from build123d import *

# Parameters (mm, degrees)
F0_W     = 40
F0_H     = 40
F1_DEPTH = 10
F2_T     = -1
F3_R     = 1.25
F4_DEPTH = 10
F5_DEPTH = 25
F6_DEPTH = 25
F7_W     = 11
F7_H     = 1
F7_W_2   = 1
F7_H_2   = 11
F8_DEPTH = 6.5


with BuildPart() as f1:
    # F0 (on Top) → F1 (new body)
    with BuildSketch(Plane.XY):
        Rectangle(F0_W, F0_H)
    extrude(amount=F1_DEPTH)

    # F2
    f2_openings = [f1.faces().sort_by_distance(p)[0] for p in [
        (0, 0, 10),
    ]]
    offset(amount=F2_T, openings=f2_openings)

    # F3 (on face) → F4 (join)
    with BuildSketch(Plane.XY):
        Polygon((-20, -8.4495466982), (-20, -20), (-10.1382084124, -20), align=None)
        with Locations((-17.6, -17.6)):
            Circle(F3_R, mode=Mode.SUBTRACT)
        Polygon((20, -8.4495466982), (10.1382084124, -20), (20, -20), align=None)
        with Locations((17.6, -17.6)):
            Circle(F3_R, mode=Mode.SUBTRACT)
        Polygon((-20, 20), (-20, 8.4495466982), (-10.1382084124, 20), align=None)
        with Locations((-17.6, 17.6)):
            Circle(F3_R, mode=Mode.SUBTRACT)
        Polygon((20, 20), (10.1382084124, 20), (20, 8.4495466982), align=None)
        with Locations((17.6, 17.6)):
            Circle(F3_R, mode=Mode.SUBTRACT)
    extrude(amount=F4_DEPTH)

    # F3 (on face) → F5 (cut)
    with BuildSketch(Plane.XY):
        with Locations((-17.6, -17.6)):
            Circle(F3_R)
        with Locations((17.6, -17.6)):
            Circle(F3_R)
        with Locations((17.6, 17.6)):
            Circle(F3_R)
        with Locations((-17.6, 17.6)):
            Circle(F3_R)
    extrude(amount=F5_DEPTH, mode=Mode.SUBTRACT)

    # F6 (cut): a face of the model
    f6_faces = [f1.faces().sort_by_distance(p)[0] for p in [
        (0, 0, 1),
    ]]
    extrude(f6_faces, amount=-F6_DEPTH, mode=Mode.SUBTRACT)

    # F7 (on face) → F8 (cut)
    with BuildSketch(Plane.XY.offset(10)):
        with Locations((0, 19.5)):
            Rectangle(F7_W, F7_H)
        with Locations((0, -19.5)):
            Rectangle(F7_W, F7_H)
        with Locations((-19.5, 0)):
            Rectangle(F7_W_2, F7_H_2)
        with Locations((19.5, 0)):
            Rectangle(F7_W_2, F7_H_2)
    extrude(amount=-F8_DEPTH, mode=Mode.SUBTRACT)


solid = f1.part
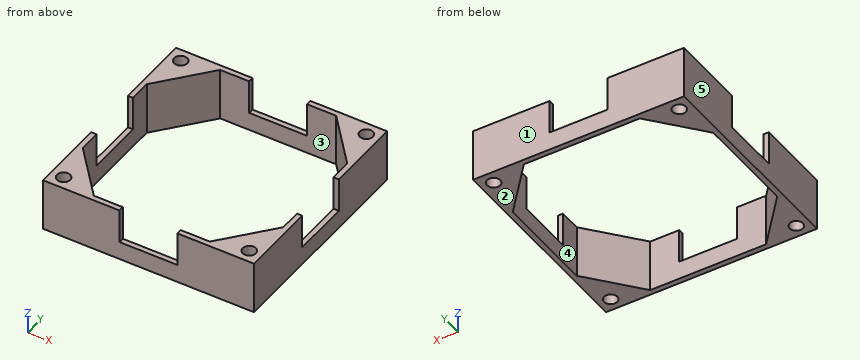
For this review, take the finished solid that the model builds, in its own axes (mm). Face numbers are marked on the shaded views. A direction names the side the tool comes from. Round coordinates to 2 decimals unless told otherwise and drop trailing zeros. Order: outer loops, then holes, each group sorted by start corner. A loop starts at its lowest first (then second) coordinate and runs counter-clockwise, first axis right, second up. Notation, with made-up numbers: M 38,-7 L 42,-7 A14 cw 42,10 Z; hole C 55.25,-28.5 d3. An arc over 180 degrees is marked long. Use a Markdown table: item, result. Add a question column.
Item 1: To check wall thickness, follow line 1 along X through (y, z) = (-3, 1.25); line 2 along Y through (x, z) = (-17, 6). State the ranges of each line that lie inside material, in increasing order.
Item 2: Add section D-D, the plane x = 17.6. Give the boundary of the cut face in (y, z), then the cut area to 3 significant figures.
Item 3: Mouldability with a two-part tool opening along Y and no side actions: class the marked faces 1, 2 and 3 as released by +Y, released by -Y, zero draft, split by the parting line, or undercut.
Item 4: Tool access review of the marked faces 4 and 5: name each direction out of +Z, -Z, +X, -X, +Y, -Y from which nothing blocks a thin tool from reaching the whole face with its end or side.
Item 5: Insertion check: pin 1 (1.1 mm diameter, centred on x = 2.5, y = -19.5, fed in from +Z); pin 2 (2 mm diameter, centred on x = -17.6, y = -17.6, fed in from -Z); pin 3 (10 mm diameter, centred on x = -13.5, y = -8.5, fed in from -Z). Each pin has a flat end and moves straight along its axis. Give the tip position at first contact, or say it passes through.
Item 6: Add section A-A, the plane z = 6. State how many separate pieces and enclosed holes the cut face has, then the cut area to 3 significant figures.
Item 7: Add section C-C, the plane y = 0.5. Give the boundary of the cut face in (x, z), then the cut area to 3 significant figures.
Item 8: Add section B-B, the plane x = -8. Give the boundary of the cut face in (y, z).
Geometry results:
| question | item | result |
|---|---|---|
| 1 | line 1 | x = -20 to -19, 19 to 20 |
| 1 | line 2 | y = -20 to -18.7, -16.5 to -11.96, 11.96 to 16.5, 18.7 to 20 |
| 2 | outline | M -20,0 L -18.85,0 L -18.85,10 L -20,10 Z; M -16.35,0 L -11.26,0 L -11.26,10 L -16.35,10 Z; M 11.26,0 L 16.35,0 L 16.35,10 L 11.26,10 Z; M 18.85,0 L 20,0 L 20,10 L 18.85,10 Z |
| 2 | area | 125 mm² |
| 3 | face 1 | released by +Y |
| 3 | face 2 | zero draft |
| 3 | face 3 | undercut |
| 4 | face 4 | +Z, -Z |
| 4 | face 5 | +Z, -Z, -X, +Y, -Y |
| 5 | pin 1 | stops at z = 3.5 |
| 5 | pin 2 | passes through |
| 5 | pin 3 | stops at z = 0 |
| 6 | separate pieces | 4 |
| 6 | enclosed holes | 4 |
| 6 | area | 243 mm² |
| 7 | outline | M -20,0 L -19,0 L -19,3.5 L -20,3.5 Z; M 19,0 L 20,0 L 20,3.5 L 19,3.5 Z |
| 7 | area | 7.00 mm² |
| 8 | outline | M -20,0 L -19,0 L -19,10 L -20,10 Z; M 19,0 L 20,0 L 20,10 L 19,10 Z |
